Work out the finished part from the listing and answer in its coordinate system (mm). A direction names the side the tool comes from. Round coordinates to 2 decimals unless told otherwise and drop trailing zeros. Write each loop counter-clockwise with the first axis right and the second up, starting at its lowest first coordinate (ties: lowest second). Pieces come first, ordered by that corner, then holes.
1. Determine the mould class of faces 3 (the face through (5.96, 1.88, 0.99)), 4 (the face through (-16.399, 15.038, 1.479)), 5 (the face through (-0.781, -8.426, 3.754)), 6 (the face through (5, -5, 0)) for opening direction X: pulls with the +X half, pulls with the -X half, needs draft (parallel to the pull), parting line crosses it, or undercut.
2. Find section C-C (z = 1.2). Write down the section's boundary in (x, y) (3 decimals).
3. A tool of negligible diameter and unlimited length cuts with its end or side. For faces 1 (the face through (-11.08, 0.15, 1.73)), 2 (the face through (3, 12, 3.5)), from which of +Z, -Z, +X, -X, +Y, -Y can it reach the whole face along a straight path? Write none if from no direction.
4. Straight lines are drawn through the part: probe 1 along Y at (x, z) = (0, 1.45) (3 decimals); probe 2 along X at (y, z) = (-1.5, 2.25); probe 3 along X at (y, z) = (3, 2.8). For each, find the intervals that lie inside material, in ascending order.
5. Find section A-A (x = 0). Write down the section's boundary in (y, z) (3 decimals).
6. Flat-ended cylindrical pins translate along their axes: pin 1 Ø4 at (x, y) = (14.375, 0) entering from -Z; pin 2 Ø11 at (x, y) = (-14.375, 0) entering from +Z. Find the tip coordinate at first contact, or state that the pin passes through.
```python
from build123d import *

# Parameters (mm, degrees)
SKETCH_1_R                   = 22.25
SKETCH_1_R_2                 = 6.25
EXTRUDE_1_DEPTH              = 4
HOLE_WIZARD_M6_1_D           = 6.6
HOLE_WIZARD_M6_1_CBORE_D     = 12
HOLE_WIZARD_M6_1_CBORE_DEPTH = 0.5
FILLET_1_R                   = 1
FILLET_2_R                   = 2


with BuildPart() as part:
    # 草图1 → 凸台-拉伸1 (new body)
    with BuildSketch(Plane.XY):
        Circle(SKETCH_1_R)
        Circle(SKETCH_1_R_2, mode=Mode.SUBTRACT)
    extrude(amount=EXTRUDE_1_DEPTH)

    # M6 六角头螺栓的柱形沉头孔1 (through all)
    with Locations(Plane.XY.offset(4)):
        with Locations((-14.375, 0), (0, 14.375), (14.375, 0), (0, -14.375)):
            CounterBoreHole(HOLE_WIZARD_M6_1_D / 2, HOLE_WIZARD_M6_1_CBORE_D / 2, HOLE_WIZARD_M6_1_CBORE_DEPTH)

    # 圆角1
    fillet_1_edges = [part.edges().sort_by_distance(p)[0] for p in [
        (-22.25, 0, 4),
    ]]
    fillet(fillet_1_edges, radius=FILLET_1_R)

    # 圆角2
    fillet_2_edges = [part.edges().sort_by_distance(p)[0] for p in [
        (-6.25, 0, 4),
    ]]
    fillet(fillet_2_edges, radius=FILLET_2_R)


solid = part.part
```
Worked answers:
1. face 3: undercut
1. face 4: parting line crosses it
1. face 5: undercut
1. face 6: needs draft
2. outline: circle Ø44.5 at (0, 0); hole circle Ø6.6 at (-14.375, 0); hole circle Ø12.5 at (0, 0); hole circle Ø6.6 at (0, -14.375); hole circle Ø6.6 at (0, 14.375); hole circle Ø6.6 at (14.375, 0)
3. face 1: +Z, -Z
3. face 2: +Z
4. probe 1: y = -22.25 to -17.675, -11.075 to -6.25, 6.25 to 11.075, 17.675 to 22.25
4. probe 2: x = -22.2 to -17.31, -11.44 to -6.08, 6.08 to 11.44, 17.31 to 22.2
4. probe 3: x = -22.05 to -15.75, -13 to -5.67, 5.67 to 13, 15.75 to 22.05
5. outline: (-22.25, 0) - (-17.675, 0) - (-17.675, 3.5) - (-20.375, 3.5) - (-20.375, 4) - (-21.25, 4) arc R1 ccw to (-22.25, 3) - close; (-11.075, 0) - (-6.25, 0) - (-6.25, 2) arc R2 ccw to (-8.25, 4) - (-8.375, 4) - (-8.375, 3.5) - (-11.075, 3.5) - close; (6.25, 0) - (11.075, 0) - (11.075, 3.5) - (8.375, 3.5) - (8.375, 4) - (8.25, 4) arc R2 ccw to (6.25, 2) - close; (17.675, 0) - (22.25, 0) - (22.25, 3) arc R1 ccw to (21.25, 4) - (20.375, 4) - (20.375, 3.5) - (17.675, 3.5) - close
6. pin 1: passes through
6. pin 2: stops at z = 3.5
